```python
from build123d import *

# Parameters (mm, degrees)
SKETCH1_R            = 1.1303
THREADS_DEPTH        = 15.875
SKETCH2_R            = 2.7559
HEAD_DEPTH           = 1.524
HEADDOME_FACE_RADIUS = 2.7559
HEADDOME_HEIGHT      = 0.508
SKETCH3_W            = 1.778
SKETCH3_H            = 1.778
DRIVER_DEPTH         = 1.524


with BuildPart() as part:
    # Sketch1 → threads (new body)
    with BuildSketch(Plane(origin=(0, 0, 0), x_dir=(1, 0, 0), z_dir=(0, 1, 0))):
        with Locations(Location((0, 0, 0), (0, 0, 270))):
            Circle(SKETCH1_R)
    extrude(amount=-THREADS_DEPTH)

    # Sketch2 → Head (add)
    with BuildSketch(Plane(origin=(0, 0, 0), x_dir=(1, 0, 0), z_dir=(0, 1, 0))):
        with Locations(Location((0, 0, 0), (0, 0, 90))):
            Circle(SKETCH2_R)
    extrude(amount=HEAD_DEPTH)

    # HeadDome: a dome of height H over a round flat face of radius A is a cap of a sphere of radius (A * A + H * H) / (2 * H)
    headdome_r = (HEADDOME_FACE_RADIUS * HEADDOME_FACE_RADIUS + HEADDOME_HEIGHT * HEADDOME_HEIGHT) / (2 * HEADDOME_HEIGHT)
    headdome_base = Plane((0, 1.524, 0), z_dir=(0, 1, 0))
    with Locations(headdome_base.offset(HEADDOME_HEIGHT - headdome_r)):
        headdome_ball = Sphere(headdome_r, mode=Mode.PRIVATE)
    add(split(headdome_ball, bisect_by=headdome_base, keep=Keep.TOP, mode=Mode.PRIVATE))

    # Sketch3 → Driver (cut)
    with BuildSketch(Plane(origin=(0, 2.032, 0), x_dir=(1, 0, 0), z_dir=(0, 1, 0))):
        Rectangle(SKETCH3_W, SKETCH3_H)
    extrude(amount=-DRIVER_DEPTH, mode=Mode.SUBTRACT)


solid = part.part
```
Geometry check sheet. Reference: the model listing, model coordinates, mm. A direction names the side the tool comes from. Give positions to 0.01 mm unless a question says otherwise; leave off trailing zeros. Write each loop counter-clockwise with the first axis right and the second up, starting at its lowest first coordinate (ties: lowest second). Pieces come first, ordered by that corner, then holes.
1) Section check A-A, the plane x = 0. Record the boundary of the cut face in (y, z) (3 decimals).
2) Material ranges on L1, parallel to Z at x = -0.7, y = -8.75; L2, parallel to X at y = -14.75, z = -0.8; L3, parallel to Y at x = -2.15, z = 0.2, recorded low to high.
3) Section check C-C, the plane y = -4.5. Record the boundary of the cut face in (x, z).
4) Section check B-B, the plane z = 0. Record the boundary of the cut face in (x, y) (3 decimals), and give its area (3 significant figures).
5) Gauge pin test, flat ends, axial feed: pin 1 (1 mm diameter, centred on x = 0, y = -1, fed in from +Z); pin 2 (0.5 mm diameter, centred on x = -0.5, z = -0.5, fed in from +Y); pin 3 (2 mm diameter, centred on x = -1, z = 1.5, fed in from +Y). Record the tip position at first contact, or that the pin passes through.
6) Access from +Z, -Z, +X, -X, +Y, -Y to the whole of each face (thin tool, end or side, straight path). Record for faces 1 (the flat face through (-0.889, 1, 0)), 2 (the cylindrical face through (-1.863, 0.751, 2.031)).
7) Release check for a two-part mould opening along X. For faces 3 (the cylindrical face through (0.34, -7.83, 1.08)), 4 (the flat face through (0, 1, -0.889)), 5 (the flat face through (1, 0, -1)) record: pulls with the +X half, pulls with the -X half, needs draft (parallel to the pull), parting line crosses it, or undercut.
8) Section check D-D, the plane z = 1.5. Record the boundary of the cut face in (x, y).
Computed:
1. outline: (-15.875, -1.13) - (0, -1.13) - (0, -2.756) - (1.524, -2.756) arc R7.729 ccw to (1.981, -0.889) - (0.508, -0.889) - (0.508, 0.889) - (1.981, 0.889) arc R7.729 ccw to (1.524, 2.756) - (0, 2.756) - (0, 1.13) - (-15.875, 1.13) - close
2. L1: z = -0.89 to 0.89
2. L2: x = -0.8 to 0.8
2. L3: y = 0 to 1.72
3. outline: circle Ø2.26 at (0, 0)
4. outline: (-2.756, 0) - (-1.13, 0) - (-1.13, -15.875) - (1.13, -15.875) - (1.13, 0) - (2.756, 0) - (2.756, 1.524) arc R7.729 ccw to (0.889, 1.981) - (0.889, 0.508) - (-0.889, 0.508) - (-0.889, 1.981) arc R7.729 ccw to (-2.756, 1.524) - close
4. area: 43.5 mm2
5. pin 1: stops at z = 1.13
5. pin 2: stops at y = 0.51
5. pin 3: stops at y = 1.98
6. face 1: +Y
6. face 2: +Y, -Y
7. face 3: parting line crosses it
7. face 4: undercut
7. face 5: needs draft
8. outline: (-2.31, 0) - (2.31, 0) - (2.31, 1.52) arc R7.58 ccw to (-2.31, 1.52) - close
